from build123d import *

# Parameters (mm, degrees)
SKETCH1_R           = 1.5
SKETCH1_R_2         = 6.5
SKETCH1_W           = 23.65
SKETCH1_H           = 42.25
BOSS_EXTRUDE1_DEPTH = 3
FILLET1_R           = 4


with BuildPart() as part:
    # Sketch1 → Boss-Extrude1 (new body)
    with BuildSketch(Plane.XY):
        Polygon((12.62, 29), (12.62, 21.5), (2.8, 21.5), (2.8, 24.5), (-7.2, 24.5), (-7.2, 21.5), (-21.2, 21.5), (-21.2, -21.5), (-7.2, -21.5), (-7.2, -24.5), (2.8, -24.5), (2.8, -21.5), (12.62, -21.5), (12.62, -29), (44.63, -29), (44.63, 29), align=None)
        with Locations((-15, -8)):
            Circle(SKETCH1_R, mode=Mode.SUBTRACT)
        with Locations((-15, 8)):
            Circle(SKETCH1_R, mode=Mode.SUBTRACT)
        with Locations((11, 12)):
            Circle(SKETCH1_R, mode=Mode.SUBTRACT)
        with Locations((11, -12)):
            Circle(SKETCH1_R, mode=Mode.SUBTRACT)
        Circle(SKETCH1_R_2, mode=Mode.SUBTRACT)
        with BuildLine():
            Line((22.229319933, 27.05), (25.229319933, 27.05))
            ThreePointArc((25.229319933, 27.05), (26.729319933, 25.55), (25.229319933, 24.05))
            Line((25.229319933, 24.05), (22.229319933, 24.05))
            ThreePointArc((22.229319933, 24.05), (20.729319933, 25.55), (22.229319933, 27.05))
        make_face(mode=Mode.SUBTRACT)
        with BuildLine():
            Line((32.029319933, 27.05), (35.029319933, 27.05))
            ThreePointArc((35.029319933, 27.05), (36.529319933, 25.55), (35.029319933, 24.05))
            Line((35.029319933, 24.05), (32.029319933, 24.05))
            ThreePointArc((32.029319933, 24.05), (30.529319933, 25.55), (32.029319933, 27.05))
        make_face(mode=Mode.SUBTRACT)
        with BuildLine():
            Line((22.229319933, -24.05), (25.229319933, -24.05))
            ThreePointArc((25.229319933, -24.05), (26.729319933, -25.55), (25.229319933, -27.05))
            Line((25.229319933, -27.05), (22.229319933, -27.05))
            ThreePointArc((22.229319933, -27.05), (20.729319933, -25.55), (22.229319933, -24.05))
        make_face(mode=Mode.SUBTRACT)
        with Locations((28.625, 0)):
            Rectangle(SKETCH1_W, SKETCH1_H, mode=Mode.SUBTRACT)
        with BuildLine():
            Line((32.029319933, -24.05), (35.029319933, -24.05))
            ThreePointArc((35.029319933, -24.05), (36.529319933, -25.55), (35.029319933, -27.05))
            Line((35.029319933, -27.05), (32.029319933, -27.05))
            ThreePointArc((32.029319933, -27.05), (30.529319933, -25.55), (32.029319933, -24.05))
        make_face(mode=Mode.SUBTRACT)
    extrude(amount=BOSS_EXTRUDE1_DEPTH)

    # Fillet1
    fillet1_edges = [part.edges().sort_by_distance(p)[0] for p in [
        (12.62, 29, 1.5),
        (44.63, 29, 1.5),
        (44.63, -29, 1.5),
        (12.62, -29, 1.5),
    ]]
    fillet(fillet1_edges, radius=FILLET1_R)


solid = part.part
Could you check a few things on this model? Use its own coordinates, in mm. A direction names the side the tool comes from. Coordinates: 2 decimals unless noted, no trailing zeros. Order: outer loops, then holes, each group sorted by start corner. A loop starts at its lowest first (then second) coordinate and runs counter-clockwise, first axis right, second up. Notation, with made-up numbers: (-6.5, 64) -> (49.5, 64) arc R31 ccw to (49.5, 89) -> close; hole circle Ø10 at (24, 31). An arc over 180 degrees is marked (long way). One line per question, with ' | ' between items.
Q1. Thinking about a two-plate mould opening in Y: for faces 1 (the face through (36.53, -25.52, 1.48)), 2 (the face through (28, -29, 1)), 3 (the face through (13.761, 27.797, 1.521)), 4 (the face through (2.8, 23, 1)), which applies, pulls with the +Y half, pulls with the -Y half, needs draft (parallel to the pull), parting line crosses it, or undercut?
Return value:
face 1: undercut | face 2: pulls with the -Y half | face 3: pulls with the +Y half | face 4: needs draft
Q2. Imagine slicing it at D-D on z = 1.6. State how many separate pieces and enclosed holes the cut face has, and give its area (3 significant figures).
Return value:
separate pieces: 1 | enclosed holes: 10 | area: 2,130 mm²
Q3. On a 3-axis mill with a long thin cutter (end or side, diameter ignored), from which of +Z, -Z, +X, -X, +Y, -Y can I reach the whole of each face in a straight line? I mean faces 5 (the face through (-14, -21.5, 1)), 6 (the face through (26.73, 25.58, 1.48)), 7 (the face through (-2, 24.5, 1)). Say none if no direction works.
Return value:
face 5: +Z, -Z, -X, -Y | face 6: +Z, -Z | face 7: +Z, -Z, -X, +Y
Q4. I'm going to push flat-ended pins straight in: P1, Ø1.5, axis at x = -3.5, z = 1.5, coming from the -Y side; P2, Ø1.5, axis at y = -23, z = 2, coming from the -X side; P3, Ø1.5, axis at x = -10.5, z = 2, coming from the +Y side. Where does each tip first touch, or does it pass through?
Return value:
P1: y = -24.5 | P2: x = -7.2 | P3: y = 21.5
Q5. Imagine slicing it at B-B on x = 11. Please give me the cut outline in (y, z), and give its area (3 significant figures).
Return value:
outline: (-21.5, 0) -> (-13.5, 0) -> (-13.5, 3) -> (-21.5, 3) -> close; (-10.5, 0) -> (10.5, 0) -> (10.5, 3) -> (-10.5, 3) -> close; (13.5, 0) -> (21.5, 0) -> (21.5, 3) -> (13.5, 3) -> close | area: 111 mm²
Q6. Imagine slicing it at C-C on y = -18. Please give me the cut outline in (x, z).
Return value:
outline: (-21.2, 0) -> (16.8, 0) -> (16.8, 3) -> (-21.2, 3) -> close; (40.45, 0) -> (44.63, 0) -> (44.63, 3) -> (40.45, 3) -> close
Q7. If I drill on L1, parallel to Y at x = -15, z = 2.25; L2, parallel to Y at x = 11, z = 1; L3, parallel to Y at x = 37, z = 0.9 (3 decimals), over which ranges is the centre line in solid material (lowest first)?
Return value:
L1: -21.5 to -9.5, -6.5 to 6.5, 9.5 to 21.5 | L2: -21.5 to -13.5, -10.5 to 10.5, 13.5 to 21.5 | L3: -29 to -21.125, 21.125 to 29
Q8. Imagine slicing it at A-A on y = -12. Please give me the cut outline in (x, z).
Return value:
outline: (-21.2, 0) -> (9.5, 0) -> (9.5, 3) -> (-21.2, 3) -> close; (12.5, 0) -> (16.8, 0) -> (16.8, 3) -> (12.5, 3) -> close; (40.45, 0) -> (44.63, 0) -> (44.63, 3) -> (40.45, 3) -> close
